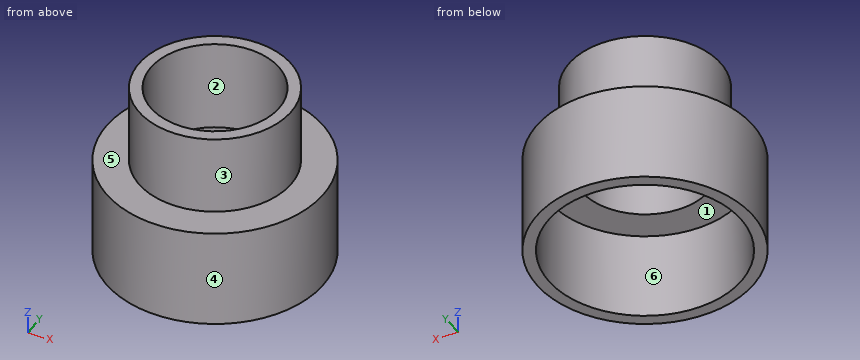
Autodesk Inventor part; units mm, degrees
ref_plane "YZ Plane" through (0, 0, 0) normal (1, 0, 0) x (0, 1, 0)
ref_plane "XZ Plane" through (0, 0, 0) normal (0, 1, 0) x (-1, 0, 0)
ref_plane "XY Plane" through (0, 0, 0) normal (0, 0, 1) x (1, 0, 0)
sketch "Sketch1" plane through (0, 0, 0) normal (0, 1, 0) x (-1, 0, 0)
  line L0 (0, 0) -> (-24.13, 0) construction
  line L1 (-24.13, 0) -> (-24.13, 22)
  line L2 (-19.05, 25) -> (-19.05, 45)
  line L3 (-24.13, 0) -> (-27.13, 0)
  line L4 (-27.13, 0) -> (-27.13, 25)
  line L5 (-27.13, 25) -> (-19.05, 25)
  line L6 (-27.13, 25) -> (-27.13, 25)
  line L7 (-27.13, 25) -> (-19.05, 25)
  line L8 (-19.05, 25) -> (-19.05, 25)
  line L9 (-19.05, 22) -> (-24.13, 22)
  line L10 (-16.05, 22) -> (-16.05, 45)
  line L11 (-19.05, 22) -> (-16.05, 22)
  line L12 (-16.05, 45) -> (-19.05, 45)
  line L13 (0, -9) -> (0, 54)
  dimension "d3" = 24.13
  dimension "d6" = 20
  dimension "d7" = 3
  dimension "d8" = 25
revolve "Revolution1" add sketch "Sketch1" angle 360 about axis through (0, 0, -10) along (0, 0, 1)
thread "Thread1"
properties part number "1-1&2 FEMALE ADAPTER"
Could you check a few things on this model? Use its own coordinates, in mm. Face numbers are marked on the shaded views. A direction names the side the tool comes from. Round coordinates to 2 decimals unless told otherwise and drop trailing zeros. Loops run counter-clockwise (first coordinate to the right, second up) from the corner with the lowest first, then second, coordinate; pieces in that order, holes last. Notation, with made-up numbers: (33.25, -7.5) - (37.25, -7.5) arc R7 cw to (37.25, -3.5) - close; hole circle Ø2 at (-2.5, 84). An arc over 180 degrees is marked (long way). Write item = value, one per line.
1) I need wall thicknesses on line 1 along Y through (x, z) = (0, 34.5); line 2 along Y through (x, z) = (0, 10.5); line 3 along Z through (x, y) = (-14, 9). Which ranges of each line are inside material? Lowest first, please. Write a range as from..to.
Computed:
line_1 = -19.05..-16.05, 16.05..19.05
line_2 = -27.13..-24.13, 24.13..27.13
line_3 = 22..45
2) Imagine slicing it at D-D (x = 21.5). Please give me the cut outline in (y, z).
Computed:
outline = (-16.55, 0) - (-10.95, 0) - (-10.95, 22) - (10.95, 22) - (10.95, 0) - (16.55, 0) - (16.55, 25) - (-16.55, 25) - close
3) On a 3-axis mill with a long thin cutter (end or side, diameter ignored), from which of +Z, -Z, +X, -X, +Y, -Y can I reach the whole of each face in a straight line? I mean the marked faces 1, 2 and 3. Say none if no direction works.
Computed:
face_1 = -Z
face_2 = +Z, -Z
face_3 = +Z
4) If we mould it in two halves opening along Y, with no side actions, what happens to the marked faces 4, 5 and 6? For each: pulls with the +Y half, pulls with the -Y half, needs draft (parallel to the pull), parting line crosses it, or undercut.
Computed:
face_4 = parting line crosses it
face_5 = needs draft
face_6 = undercut
5) Imagine slicing it at A-A (y = 0). Please give me the cut outline in (x, z), and give its area (3 significant figures).
Computed:
outline = (-27.13, 0) - (-24.13, 0) - (-24.13, 22) - (-16.05, 22) - (-16.05, 45) - (-19.05, 45) - (-19.05, 25) - (-27.13, 25) - close; (16.05, 22) - (24.13, 22) - (24.13, 0) - (27.13, 0) - (27.13, 25) - (19.05, 25) - (19.05, 45) - (16.05, 45) - close
area = 318 mm2
6) I'm going to push flat-ended pins straight in: P1, Ø12, axis at y = 0.5, z = 14, coming from the +X side; P2, Ø10, axis at y = -14, z = 26, coming from the -X side; P3, Ø1.5, axis at x = -11.5, z = 6.5, coming from the +Y side; P4, Ø14.5, axis at x = -3.5, y = -8, coming from the -Z side. Where does each tip first touch, or does it pass through?
Computed:
P1 = 27.13
P2 = -25.56
P3 = 24.91
P4 = through
7) Imagine slicing it at C-C (z = 37). Please give me the cut outline in (x, y).
Computed:
outline = circle Ø38.1 at (0, 0); hole circle Ø32.1 at (0, 0)
